Build history of the part. All positions in model axes, mm. A direction names the side the tool comes from. Give positions to 0.01 mm unless a question says otherwise; leave off trailing zeros. Write each loop counter-clockwise with the first axis right and the second up, starting at its lowest first coordinate (ties: lowest second). Pieces come first, ordered by that corner, then holes. Notation, with made-up numbers: M 84,77.25 L 123,77.25 A21 cw 123,81.25 Z; hole C 48.25,84.25 d8. An arc over 180 degrees is marked long. Return JSON: item names as keys, results as strings. Group by question number.
Q1. Band-saw the part on A-A, the plane y = -22. Give the cut face in (x, z).
Q2. Flat gauge pins, fed straight in: pin 1 Ø6 at (x, y) = (-28.36, 26.26) entering from +Z; pin 2 Ø8 at (x, y) = (13, 11) entering from +Z; pin 3 Ø4.5 at (x, y) = (18, 26) entering from -Z. Where does each tip first touch, or does it go through?
Q3. Wall check: probe 1 along Z at (x, y) = (-4.5, 26); probe 2 along Z at (x, y) = (-16, 2); probe 3 along Y at (x, z) = (-27.5, 40). Give the ranges that are in metal, low to high.
Q4. Tool access for faces 1 (the cylindrical face through (22.213, -14.232, 25.35)), 2 (the cylindrical face through (-31.94, -14.23, 25.35)), 3 (the cylindrical face through (12.135, 29.838, 25.35)): list every direction of +Z, -Z, +X, -X, +Y, -Y with a clear straight run to the whole face (end or side of a thin tool).
Q5. Band-saw the part on C-C, the plane x = 3.5. Give the cut face in (y, z), then the cut area to 3 significant figures.
Q6. Band-saw the part on D-D, the plane y = 1.5. Give the cut face in (x, z).
from build123d import *

# Parameters (mm, degrees)
SKETCH1_W            = 57
SKETCH1_H            = 57
BOSS_EXTRUDE1_DEPTH  = 55
SKETCH2_W            = 10
SKETCH2_H            = 10
CUT_EXTRUDE1_DEPTH   = 50
LPATTERN1_COUNT      = 2
LPATTERN1_PITCH      = 47
LPATTERN1_COUNT_DIR2 = 2
LPATTERN1_PITCH_DIR2 = 47
SKETCH3_R            = 2.5
CUT_EXTRUDE2_DEPTH   = 50
LPATTERN2_COUNT      = 2
LPATTERN2_PITCH      = 47
LPATTERN2_COUNT_DIR2 = 2
LPATTERN2_PITCH_DIR2 = 47
FILLET1_R            = 5
SKETCH5_R            = 19.05
BOSS_EXTRUDE3_DEPTH  = 1.5
SKETCH4_R            = 4
BOSS_EXTRUDE2_DEPTH  = 28.5


with BuildPart() as part:
    # Sketch1 → Boss-Extrude1 (new body)
    with BuildSketch(Plane.XY):
        with Locations((-4.861204013, 2.764214047)):
            Rectangle(SKETCH1_W, SKETCH1_H)
    extrude(amount=BOSS_EXTRUDE1_DEPTH)

    # Sketch2 → Cut-Extrude1 (cut)
    with BuildSketch(Plane(origin=(0, 0, 0), x_dir=(-1, 0, 0), z_dir=(0, 0, -1))):
        with Locations((-18.638795987, 26.264214047)):
            Rectangle(SKETCH2_W, SKETCH2_H)
    cut_extrude1 = extrude(amount=-CUT_EXTRUDE1_DEPTH, mode=Mode.SUBTRACT)

    # LPattern1: Cut-Extrude1 2 × 2
    with Locations(*[(-i * LPATTERN1_PITCH, -j * LPATTERN1_PITCH_DIR2, 0) for i in range(LPATTERN1_COUNT) for j in range(LPATTERN1_COUNT_DIR2) if (i, j) != (0, 0)]):
        add(cut_extrude1, mode=Mode.SUBTRACT)

    # Sketch3 → Cut-Extrude2 (cut)
    with BuildSketch(Plane.XY.offset(55)):
        with Locations((-28.361204013, 26.264214047)):
            Circle(SKETCH3_R)
    cut_extrude2 = extrude(amount=-CUT_EXTRUDE2_DEPTH, mode=Mode.SUBTRACT)

    # LPattern2: Cut-Extrude2 2 × 2
    with Locations(*[(i * LPATTERN2_PITCH, -j * LPATTERN2_PITCH_DIR2, 0) for i in range(LPATTERN2_COUNT) for j in range(LPATTERN2_COUNT_DIR2) if (i, j) != (0, 0)]):
        add(cut_extrude2, mode=Mode.SUBTRACT)

    # Fillet1
    fillet1_edges = [part.edges().sort_by_distance(p)[0] for p in [
        (-33.361204013, 21.264214047, 25),
        (-23.361204013, 21.264214047, 25),
        (-23.361204013, 31.264214047, 25),
        (13.638795987, 31.264214047, 25),
        (13.638795987, 21.264214047, 25),
        (23.638795987, 21.264214047, 25),
        (23.638795987, -25.735785953, 52.5),
        (23.638795987, -15.735785953, 25),
        (13.638795987, -15.735785953, 25),
        (13.638795987, -25.735785953, 25),
        (-23.361204013, -25.735785953, 25),
        (-23.361204013, -15.735785953, 25),
        (-33.361204013, -15.735785953, 25),
        (-33.361204013, -25.735785953, 52.5),
        (-33.361204013, 31.264214047, 52.5),
        (23.638795987, 31.264214047, 52.5),
    ]]
    fillet(fillet1_edges, radius=FILLET1_R - 0.0001)  # a hair under: the kernel refuses the full size

    # Sketch5 → Boss-Extrude3 (add)
    with BuildSketch(Plane.XY.offset(55)):
        with Locations((-4.861204013, 2.764214047)):
            Circle(SKETCH5_R)
    extrude(amount=BOSS_EXTRUDE3_DEPTH)

    # Sketch4 → Boss-Extrude2 (add)
    with BuildSketch(Plane.XY.offset(55)):
        with Locations(Location((-4.861204013, 2.764214047, 0), (0, 0, 180))):
            Circle(SKETCH4_R)
    extrude(amount=BOSS_EXTRUDE2_DEPTH)


solid = part.part
From the geometry:
{
 "1": {"outline": "M -33.2,50 L -30.52,50 L -30.52,55 L -33.2,55 Z; M -26.2,50 L -23.2,50 L -23.2,0 L 13.48,0 L 13.48,50 L 16.48,50 L 16.48,55 L -26.2,55 Z; M 20.8,50 L 23.48,50 L 23.48,55 L 20.8,55 Z"},
 "2": {"pin 1": "stops at z = 55", "pin 2": "stops at z = 56.5", "pin 3": "stops at z = 50"},
 "3": {"probe 1": "z = 0 to 55", "probe 2": "z = 0 to 56.5", "probe 3": "y = -15.81 to 21.34"},
 "4": {"face 1": "-Z, +X, -Y", "face 2": "-Z, -X, -Y", "face 3": "-Z, +X, +Y"},
 "5": {"outline": "M -25.74,0 L 31.26,0 L 31.26,55 L 19.88,55 L 19.88,56.5 L -14.35,56.5 L -14.35,55 L -25.74,55 Z", "area": "3,190 mm^2"},
 "6": {"outline": "M -33.36,0 L 23.64,0 L 23.64,55 L 14.15,55 L 14.15,56.5 L -1.07,56.5 L -1.07,83.5 L -8.66,83.5 L -8.66,56.5 L -23.87,56.5 L -23.87,55 L -33.36,55 Z"}
}
